Verification items for the finished model (mm, model axes). Face numbers are marked on the shaded views. A direction names the side the tool comes from. Coordinates: 2 decimals unless noted, no trailing zeros. Order: outer loops, then holes, each group sorted by start corner. A loop starts at its lowest first (then second) coordinate and runs counter-clockwise, first axis right, second up. Notation, with made-up numbers: M 60,49.25 L 81,49.25 A20 ccw 81,71.25 Z; hole C 76.25,28 d6. An arc over 180 degrees is marked long. Return JSON: item names as keys, results as strings. Group by question number.
Q1. Mould release check, pull along Z, two halves, no side actions. Record for the marked faces 3, 4, 5 and 6: pulls with the +Z half, pulls with the -Z half, needs draft (parallel to the pull), parting line crosses it, or undercut.
Q2. Access from +Z, -Z, +X, -X, +Y, -Y to the whole of each face (thin tool, end or side, straight path). Record for the marked faces 1 and 2.
Q3. Thickness scan on probe 1 along Z at (x, y) = (0, 1.15); probe 2 along Y at (x, z) = (-1.25, -6.5); probe 3 along Z at (x, y) = (0, -1.15). Record the ranges inside material, lowest first.
Q4. Section check C-C, the plane x = 0. Enter the section's corners in (y, z).
Q5. Section check B-B, the plane y = 0.4. Enter the section's corners in (x, z).
Q6. Section check A-A, the plane z = 0. Enter the section's corners in (x, y), then the cut area to 3 significant figures.
Q7. Go/stop test with flat-tipped pins: pin 1 Ø1.5 at (x, y) = (-4, 1) entering from -Z; pin 2 Ø1.5 at (x, y) = (0, 1) entering from +Z; pin 3 Ø2 at (x, y) = (1.5, -1.5) entering from -Z; pin 4 Ø1.5 at (y, z) = (-0.5, -5) entering from +X. Record where each tip stops, or that it passes through.
Q8. Section check D-D, the plane y = -0.7. Enter the section's corners in (x, z).
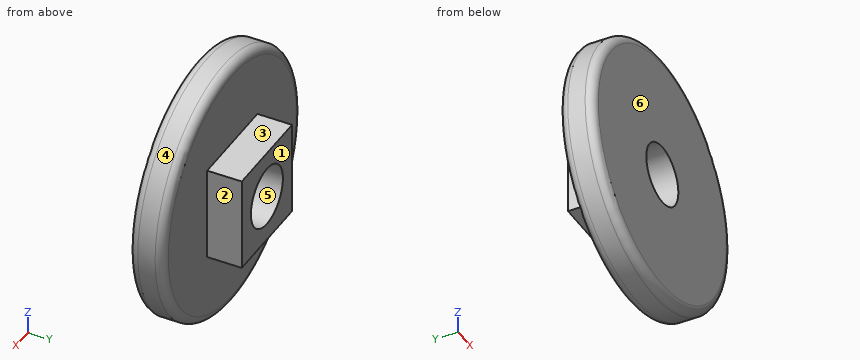
Autodesk Inventor part; units mm, degrees
ref_plane "YZ Plane" through (0, 0, 0) normal (1, 0, 0) x (0, 1, 0)
ref_plane "XZ Plane" through (0, 0, 0) normal (0, 1, 0) x (-1, 0, 0)
ref_plane "XY Plane" through (0, 0, 0) normal (0, 0, 1) x (1, 0, 0)
sketch "Sketch1" plane through (0, 0, 0) normal (0, 1, 0) x (-1, 0, 0)
  circle A0 centre (0, 0) radius 1.75
  circle A1 centre (0, 0) radius 7.5
  line L0 (-2.75, -2.75) -> (2.75, -2.75)
  line L1 (2.75, -2.75) -> (2.75, 2.75)
  line L2 (2.75, 2.75) -> (-2.75, 2.75)
  line L3 (-2.75, 2.75) -> (-2.75, -2.75)
  line L4 (-2.75, -2.75) -> (2.75, 2.75) construction
  line L5 (2.75, -2.75) -> (-2.75, 2.75) construction
  dimension "d1" = 3.5
  dimension "d2" = 15
  dimension "d3" = 5.5
  dimension "d4" = 5.5
extrude "Extrusion1" add sketch "Sketch1" along normal blind 2 contours L3 L2 L1 L0
extrude "Extrusion2" add sketch "Sketch1" against normal blind 2 contours A1 | L3 L2 L1 L0
fillet "Fillet1" radius 0.5 2 edges at (7.5, 0, 0) (7.5, -2, 0)
equation "\"d2\" = CapDiameter"
equation "\"d5\" = PIVOT_DEPTH"
equation "\"d7\" = CapHeight"
equation "\"CapDiameter\" = 15"
equation "\"CapHeight\" = 2"
properties part number "FrictionCap"
Numbers:
{
 "1": {"face 3": "pulls with the +Z half", "face 4": "parting line crosses it", "face 5": "undercut", "face 6": "needs draft"},
 "2": {"face 1": "+Z, -Z, +X, -X, +Y", "face 2": "+Z, -Z, +X, +Y"},
 "3": {"probe 1": "z = -2.75 to -1.75, 1.75 to 2.75", "probe 2": "y = -2 to 0", "probe 3": "z = -7.5 to -1.75, 1.75 to 7.5"},
 "4": {"outline": "M -2,-7 A0.5 ccw -1.5,-7.5 L -0.5,-7.5 A0.5 ccw 0,-7 L 0,-2.75 L 2,-2.75 L 2,-1.75 L -2,-1.75 Z; M -2,1.75 L 2,1.75 L 2,2.75 L 0,2.75 L 0,7 A0.5 ccw -0.5,7.5 L -1.5,7.5 A0.5 ccw -2,7 Z"},
 "5": {"outline": "M -2.75,-2.75 L 2.75,-2.75 L 2.75,2.75 L -2.75,2.75 Z; hole C 0,0 d3.5"},
 "6": {"outline": "M -7.5,-1.5 A0.5 ccw -7,-2 L -1.75,-2 L -1.75,2 L -2.75,2 L -2.75,0 L -7,0 A0.5 ccw -7.5,-0.5 Z; M 1.75,-2 L 7,-2 A0.5 ccw 7.5,-1.5 L 7.5,-0.5 A0.5 ccw 7,0 L 2.75,0 L 2.75,2 L 1.75,2 Z", "area": "26.8 mm2"},
 "7": {"pin 1": "passes through", "pin 2": "stops at z = 2.75", "pin 3": "stops at z = -7.48", "pin 4": "stops at x = 6.18"},
 "8": {"outline": "C 0,0 d15; hole C 0,0 d3.5"}
}
